```python
from build123d import *

# Parameters (mm, degrees)
SKETCH_1_W                           = 57
SKETCH_1_H                           = 57
EXTRUDE_1_DEPTH                      = 4.5
FILLET_1_R                           = 5
SKETCH_2_R                           = 25.1
CUT_EXTRUDE_1_DEPTH                  = 3
SKETCH_3_R                           = 23.5
CUT_EXTRUDE_2_DEPTH                  = 1.5
SKETCH_4_R                           = 2.5
SKETCH_4_R_2                         = 1.7
CUT_EXTRUDE_3_DEPTH                  = 41.555517504
EXTRUDE_2_DEPTH                      = 1
CHAMFER_1_SIZE                       = 0.2
CUT_EXTRUDE_4_DEPTH                  = 1.1
PATTERN_CIRCULAR_1_COUNT             = 4
CHAMFER_1_OF_PATTERN_CIRCULAR_1_SIZE = 0.2


with BuildPart() as part:
    # 草图1 → 凸台-拉伸1 (new body)
    with BuildSketch(Plane(origin=(0, 0, 0), x_dir=(1, 0, 0), z_dir=(0, 1, 0))):
        Rectangle(SKETCH_1_W, SKETCH_1_H)
    extrude(amount=EXTRUDE_1_DEPTH)

    # 圆角1
    fillet_1_edges = [part.edges().sort_by_distance(p)[0] for p in [
        (28.5, 2.25, 28.5),
        (-28.5, 2.25, 28.5),
        (-28.5, 2.25, -28.5),
        (28.5, 2.25, -28.5),
    ]]
    fillet(fillet_1_edges, radius=FILLET_1_R)

    # 草图2 → 切除-拉伸1 (cut)
    with BuildSketch(Plane(origin=(0, 4.5, 0), x_dir=(1, 0, 0), z_dir=(0, 1, 0))):
        with Locations(Location((0, 0, 0), (0, 0, 270))):
            Circle(SKETCH_2_R)
    extrude(amount=-CUT_EXTRUDE_1_DEPTH, mode=Mode.SUBTRACT)

    # 草图3 → 切除-拉伸2 (cut)
    with BuildSketch(Plane(origin=(0, 1.5, 0), x_dir=(1, 0, 0), z_dir=(0, 1, 0))):
        with Locations(Location((0, 0, 0), (0, 0, 270))):
            Circle(SKETCH_3_R)
    extrude(amount=-CUT_EXTRUDE_2_DEPTH, mode=Mode.SUBTRACT)

    # 草图4 → 切除-拉伸3 (cut, through all)
    with BuildSketch(Plane(origin=(0, 4.5, 0), x_dir=(1, 0, 0), z_dir=(0, 1, 0))):
        with Locations(Location((-23.5, 23.5, 0), (0, 0, 270))):
            Circle(SKETCH_4_R)
        with Locations(Location((-15.5, 25, 0), (0, 0, 270))):
            Circle(SKETCH_4_R_2)
    cut_extrude_3 = extrude(amount=-CUT_EXTRUDE_3_DEPTH, mode=Mode.SUBTRACT)

    # 草图5 → 凸台-拉伸2 (add)
    with BuildSketch(Plane(origin=(0, 4.5, 0), x_dir=(1, 0, 0), z_dir=(0, 1, 0))):
        Polygon((-28.5, 11), (-28.5, -11), (-27.5, -10), (-27.5, 10), align=None)
    extrude_2 = extrude(amount=EXTRUDE_2_DEPTH)

    # 倒角1
    chamfer_1_edges = [part.edges().sort_by_distance(p)[0] for p in [
        (-27.5, 5.5, 0),
    ]]
    chamfer(chamfer_1_edges, length=CHAMFER_1_SIZE)

    # 草图6 → 切除-拉伸4 (cut)
    with BuildSketch(Plane.XZ):
        Polygon((-28.5, 11.1), (-28.5, -11.1), (-27.5, -10.1), (-27.5, 10.1), align=None)
    cut_extrude_4 = extrude(amount=-CUT_EXTRUDE_4_DEPTH, mode=Mode.SUBTRACT)

    # 阵列(圆周)1: 切除-拉伸3, 凸台-拉伸2, 切除-拉伸4 ×4 about axis
    pattern_circular_1_axis = Axis((0, 0, 0), (0, 1, 0))
    add([cut_extrude_3.rotate(pattern_circular_1_axis, i * 360 / PATTERN_CIRCULAR_1_COUNT) for i in range(1, PATTERN_CIRCULAR_1_COUNT)], mode=Mode.SUBTRACT)
    add([extrude_2.rotate(pattern_circular_1_axis, i * 360 / PATTERN_CIRCULAR_1_COUNT) for i in range(1, PATTERN_CIRCULAR_1_COUNT)])
    add([cut_extrude_4.rotate(pattern_circular_1_axis, i * 360 / PATTERN_CIRCULAR_1_COUNT) for i in range(1, PATTERN_CIRCULAR_1_COUNT)], mode=Mode.SUBTRACT)

    # 倒角1 of 阵列(圆周)1
    chamfer_1_of_pattern_circular_1_edges = [part.edges().sort_by_distance(p)[0] for p in [
        (0, 5.5, 27.5),
        (27.5, 5.5, 0),
        (0, 5.5, -27.5),
    ]]
    chamfer(chamfer_1_of_pattern_circular_1_edges, length=CHAMFER_1_OF_PATTERN_CIRCULAR_1_SIZE)


solid = part.part
```
Input: part model. Units: mm. Frame: model coordinates. A direction names the side the tool comes from. Give positions to 0.01 mm unless a question says otherwise; leave off trailing zeros. Order: outer loops, then holes, each group sorted by start corner. A loop starts at its lowest first (then second) coordinate and runs counter-clockwise, first axis right, second up. Notation, with made-up numbers: (-31, 62.5) -> (14, 62.5) arc R15 ccw to (14, 81.5) -> close; hole circle Ø5 at (63, -34). An arc over 180 degrees is marked (long way). Write each question's results on one line, items separated by ' | '. Start each with the question number.
Item 1: Mould query, pull axis X, two halves, no side actions, for faces 1 (the cylindrical face through (13.814, 2.282, 25.221)), 2 (the cylindrical face through (27.07, 2.28, -27)), 3 (the cylindrical face through (-27.07, 2.28, -27)), 4 (the cylindrical face through (21.81, 2.28, 25.34)). Classes: pulls with the +X half, pulls with the -X half, needs draft (parallel to the pull), parting line crosses it, or undercut.
Item 2: Line query: line 1 (X direction, y = 2.35, z = 0); line 2 (X direction, y = 0.6, z = 0); line 3 (Z direction, x = -22, y = 2.25). Output: solid intervals per line, ascending.
Item 3: Cut plane B-B on x = -6. Return the cut outline in (y, z), then the cut area to 3 significant figures.
Item 4: Set-up query: faces 5 (the flat face through (22.4, 1.5, -7.6)), 6 (the cylindrical face through (-27.07, 2.28, 27)). Return all of +Z, -Z, +X, -X, +Y, -Y with unobstructed straight access to the full face (end or side cutting, diameter ignored); none if empty.
Item 5: Cut plane A-A on z = 0. Return the cut outline in (x, y), then the cut area to 3 significant figures.
Item 6: Cut plane D-D on x = -22. Return the cut outline in (y, z), then the cut area to 3 significant figures.
Item 7: Contact query for flat-ended pins moving along their axis: P1, Ø0.9, axis at y = 0.5, z = 0, coming from the -X side; P2, Ø0.8, axis at x = -5.5, z = 28, coming from the -Y side; P3, Ø5.5, axis at x = 25, z = -15.5, coming from the +Y side. Output: stop coordinate, or through.
Item 8: Cut plane C-C on y = 2.3. Give the number of separate pieces and of enclosed holes in the cut face, then the cut area to 3 significant figures.
Established:
1) face 1: undercut | face 2: pulls with the +X half | face 3: pulls with the -X half | face 4: undercut
2) line 1: -28.5 to -25.1, 25.1 to 28.5 | line 2: -27.5 to -23.5, 23.5 to 27.5 | line 3: -28.5 to -25.5, -21.5 to -12.08, 12.08 to 21.5, 25.5 to 28.5
3) outline: (0, -27.5) -> (1.1, -27.5) -> (1.1, -28.5) -> (5.5, -28.5) -> (5.5, -27.7) -> (5.3, -27.5) -> (4.5, -27.5) -> (4.5, -24.37) -> (1.5, -24.37) -> (1.5, -22.72) -> (0, -22.72) -> close; (0, 22.72) -> (1.5, 22.72) -> (1.5, 24.37) -> (4.5, 24.37) -> (4.5, 27.5) -> (5.3, 27.5) -> (5.5, 27.7) -> (5.5, 28.5) -> (1.1, 28.5) -> (1.1, 27.5) -> (0, 27.5) -> close | area: 41.9 mm^2
4) face 5: +Y | face 6: +Z, -X, +Y, -Y
5) outline: (-28.5, 1.1) -> (-27.5, 1.1) -> (-27.5, 0) -> (-23.5, 0) -> (-23.5, 1.5) -> (-25.1, 1.5) -> (-25.1, 4.5) -> (-27.5, 4.5) -> (-27.5, 5.3) -> (-27.7, 5.5) -> (-28.5, 5.5) -> close; (23.5, 0) -> (27.5, 0) -> (27.5, 1.1) -> (28.5, 1.1) -> (28.5, 5.5) -> (27.7, 5.5) -> (27.5, 5.3) -> (27.5, 4.5) -> (25.1, 4.5) -> (25.1, 1.5) -> (23.5, 1.5) -> close | area: 35.2 mm^2
6) outline: (0, -28.5) -> (4.5, -28.5) -> (4.5, -25.5) -> (0, -25.5) -> close; (0, -21.5) -> (4.5, -21.5) -> (4.5, -12.08) -> (1.5, -12.08) -> (1.5, -8.26) -> (0, -8.26) -> close; (0, 8.26) -> (1.5, 8.26) -> (1.5, 12.08) -> (4.5, 12.08) -> (4.5, 21.5) -> (0, 21.5) -> close; (0, 25.5) -> (4.5, 25.5) -> (4.5, 28.5) -> (0, 28.5) -> close | area: 123 mm^2
7) P1: x = -27.5 | P2: y = 1.1 | P3: y = 4.5
8) separate pieces: 1 | enclosed holes: 9 | area: 1,130 mm^2
